Source: CAD feature listing. Evaluate the final solid. Frame: model axes, mm. A direction names the side the tool comes from. Give positions to 0.01 mm unless a question says otherwise; leave off trailing zeros. Loops run counter-clockwise (first coordinate to the right, second up) from the corner with the lowest first, then second, coordinate; pieces in that order, holes last.
from build123d import *

# Parameters (mm, degrees)
F1_DEPTH = 47.625
F2_R     = 7.9375
F3_DEPTH = 114.301


with BuildPart() as f1:
    # F0 (on Top) → F1 (new body, symmetric)
    with BuildSketch(Plane.XY):
        with BuildLine():
            ThreePointArc((0, 31.75), (31.75, 0), (0, -31.75))
            ThreePointArc((0, -31.75), (-12.7, -44.45), (0, -57.15))
            ThreePointArc((0, -57.15), (40.4111525448, -40.4111525448), (57.15, 0))
            Line((57.15, 0), (57.15, 31.75))
            Line((57.15, 31.75), (127, 31.75))
            Line((127, 31.75), (127, 57.15))
            Line((127, 57.15), (64.5130766445, 57.15))
            Line((64.5130766445, 57.15), (53.8438755383, 63.5))
            Line((53.8438755383, 63.5), (-113.2848898665, 63.5))
            Line((-113.2848898665, 63.5), (-124.0183680439, 57.15))
            Line((-124.0183680439, 57.15), (-196.85, 57.15))
            Line((-196.85, 57.15), (-196.85, 31.75))
            Line((-196.85, 31.75), (-133.35, 31.75))
            Line((-133.35, 31.75), (-133.35, -53.1049028658))
            Line((-133.35, -53.1049028658), (-90.5046517968, -53.1049028658))
            Line((-90.5046517968, -53.1049028658), (-90.5046517968, -31.75))
            Line((-90.5046517968, -31.75), (-107.95, -31.75))
            Line((-107.95, -31.75), (-107.95, 27.6119898381))
            Line((-107.95, 27.6119898381), (0, 27.6119898381))
            Line((0, 27.6119898381), (0, 31.75))
        make_face()
    extrude(amount=F1_DEPTH, both=True)

    # F2 (on face) → F3 (cut, through all)
    with BuildSketch(Plane(origin=(0, 57.15, 0), x_dir=(-1, 0, 0), z_dir=(0, 1, 0))):
        with Locations((-98.425, 0)):
            Circle(F2_R)
        with Locations((168.275, 0)):
            Circle(F2_R)
    extrude(amount=-F3_DEPTH, mode=Mode.SUBTRACT)


solid = f1.part
1) Pull-direction query (X, two-part tool) for faces 6 (the flat face through (-37, 31, -47.625)), 7 (the cylindrical face through (39.964, -40.853, 0.667)), 8 (the flat face through (-90.505, -43, 1)), 9 (the cylindrical face through (-12.697, -44.171, 0.667)); classes: released by +X, released by -X, zero draft, split by the parting line, or undercut.
Checks:
face 6: zero draft
face 7: released by +X
face 8: undercut
face 9: undercut
2) Cut plane C-C (x = 22.5). Return loops of the section in (y, z) (3 decimals).
Checks:
outline: (-52.534, -47.625) - (-22.401, -47.625) - (-22.401, 47.625) - (-52.534, 47.625) - close; (22.401, -47.625) - (63.5, -47.625) - (63.5, 47.625) - (22.401, 47.625) - close
3) Contact query for flat-ended pins moving along their axis: P1, Ø3, axis at y = -24, z = 12, coming from the -X side; P2, Ø10, axis at y = -5.5, z = -16, coming from the +X side; P3, Ø20.5, axis at x = 98.425, z = 0, coming from the -Y side; P4, Ø9.5, axis at x = -168.275, z = 0, coming from the -Y side. Output: stop coordinate, or through.
Checks:
P1: stops at x = -133.35
P2: stops at x = 57.15
P3: stops at y = 31.75
P4: passes through
4) Ray query, probe 1 along Y at (x, z) = (-93.5, 22); probe 2 along Y at (x, z) = (1.5, -39); probe 3 along Y at (x, z) = (112.5, 18). Return the intervals inside material, ascending.
Checks:
probe 1: y = -53.1 to -31.75, 27.61 to 63.5
probe 2: y = -57.13 to -31.71, 31.71 to 63.5
probe 3: y = 31.75 to 57.15
5) Cut plane D-D (z = -18.5). Return loops of the section in (x, y), and give its area (3 significant figures).
Checks:
outline: (-196.85, 31.75) - (-133.35, 31.75) - (-133.35, -53.1) - (-90.5, -53.1) - (-90.5, -31.75) - (-107.95, -31.75) - (-107.95, 27.61) - (0, 27.61) - (0, 31.75) arc R31.75 cw to (0, -31.75) arc R12.7 ccw to (0, -57.15) arc R57.15 ccw to (57.15, 0) - (57.15, 31.75) - (127, 31.75) - (127, 57.15) - (64.51, 57.15) - (53.84, 63.5) - (-113.28, 63.5) - (-124.02, 57.15) - (-196.85, 57.15) - close
area: 15,400 mm2
6) Reachability of faces 1 (the flat face through (89, 57.15, 1)), 2 (the flat face through (-158, 31.75, 1)), 3 (the flat face through (57.15, 16, 1)), 4 (the flat face through (-160, 57.15, 1)), 5 (the flat face through (-99, -31.75, 1)) from +Z, -Z, +X, -X, +Y, -Y: full face, straight path, thin tool, end or side. Return the list, or none.
Checks:
face 1: +Z, -Z, +X, +Y
face 2: +Z, -Z, -X, -Y
face 3: +Z, -Z, +X, -Y
face 4: +Z, -Z, -X, +Y
face 5: +Z, -Z
7) Cut plane B-B (y = -44.45). Return loops of the section in (x, z) (3 decimals), and give its area (3 significant figures).
Checks:
outline: (-133.35, -47.625) - (-90.505, -47.625) - (-90.505, 47.625) - (-133.35, 47.625) - close; (-12.7, -47.625) - (35.921, -47.625) - (35.921, 47.625) - (-12.7, 47.625) - close
area: 8,710 mm2
8) Cut plane A-A (z = 0). Return loops of the section in (x, y), and give its area (3 significant figures).
Checks:
outline: (-196.85, 31.75) - (-176.21, 31.75) - (-176.21, 57.15) - (-196.85, 57.15) - close; (-160.34, 31.75) - (-133.35, 31.75) - (-133.35, -53.1) - (-90.5, -53.1) - (-90.5, -31.75) - (-107.95, -31.75) - (-107.95, 27.61) - (0, 27.61) - (0, 31.75) arc R31.75 cw to (0, -31.75) arc R12.7 ccw to (0, -57.15) arc R57.15 ccw to (57.15, 0) - (57.15, 31.75) - (90.49, 31.75) - (90.49, 57.15) - (64.51, 57.15) - (53.84, 63.5) - (-113.28, 63.5) - (-124.02, 57.15) - (-160.34, 57.15) - close; (106.36, 31.75) - (127, 31.75) - (127, 57.15) - (106.36, 57.15) - close
area: 14,600 mm2
